The listing builds one solid part. Answer for the finished solid, in the listing's coordinates (mm). A direction names the side the tool comes from. Coordinates: 2 decimals unless noted, no trailing zeros. Loops run counter-clockwise (first coordinate to the right, second up) from the corner with the lowest first, then second, coordinate; pieces in that order, holes last. Notation, with made-up numbers: (42.25, 12.25) - (65.25, 12.25) arc R19 ccw to (65.25, 31.25) - close; hole circle Ø4 at (62, 44.25). An arc over 180 degrees is marked (long way). Return JSON: item names as keys, results as strings. Group by question number.
1. Section A-A (x = 125) is taken. Write down the section's boundary in (y, z) (3 decimals), and give its area (3 significant figures).
2. Find the intervals of material crossed by line 1 along X through (y, z) = (4.5, 0.75); line 2 along X through (y, z) = (-2.5, 0.75); line 3 along Y through (x, z) = (199, 0.25), in increasing order.
3. Which of the six approach directions +Z, -Z, +X, -X, +Y, -Y give full straight-line access (tool end or side, diameter ignored) to faces 1 (the face through (119.257, -4.588, 4.207)), 2 (the face through (22.92, -0.388, 2.955)), 3 (the face through (163.7, -0.1, -4.1))?
4. Each of these flat-tipped pins is pushed along its axis until it touches: P1, Ø2, axis at y = -5, z = -4.5, coming from the -X side; P2, Ø3, axis at x = 140, z = 3, coming from the +Y side; P3, Ø2, axis at x = 34, y = 4.5, coming from the +Z side; P4, Ø3, axis at x = 106, z = 0.5, coming from the +Y side. Where does it stop, or does it pass through?
5. The mould has two halves that part along X. Classify faces 4 (the face through (136.814, -3.135, -2.404)), 5 (the face through (69.702, -3.135, -2.404)), 6 (the face through (231.5, 3, 1)), 7 (the face through (260.162, -0.388, 2.955)): pulls with the +X half, pulls with the -X half, needs draft (parallel to the pull), parting line crosses it, or undercut.
```python
from build123d import *


with BuildPart() as part:
    # Esquisse1 → Révolution1 (revolve)
    with BuildSketch(Plane.XY):
        Polygon((0, 0), (0, 2.98), (1.7, 2.98), (1.7, 2.35), (3.4, 2.35), (3.4, 2.98), (41.9, 2.98), (41.9, 6.225), (65.9, 6.225), (65.9, 3.95), (73.4, 3.95), (73.4, 6.225), (97.4, 6.225), (97.4, 3.95), (109.7, 3.95), (109.7, 6.225), (128.55, 6.225), (128.55, 3.95), (144.85, 3.95), (144.85, 6.225), (163.7, 6.225), (163.7, 3.95), (176, 3.95), (176, 6.225), (200, 6.225), (200, 3.95), (207.5, 3.95), (207.5, 6.225), (231.5, 6.225), (231.5, 2.98), (257.6, 2.98), (257.6, 2.35), (259.3, 2.35), (259.3, 2.98), (261, 2.98), (261, 0), align=None)
    revolve(axis=Axis((0, 0, 0), (1, 0, 0)))


solid = part.part
```
The answers:
{
 "1": {"outline": "circle Ø12.45 at (0, 0)", "area": "122 mm2"},
 "2": {"line 1": "x = 41.9 to 65.9, 73.4 to 97.4, 109.7 to 128.55, 144.85 to 163.7, 176 to 200, 207.5 to 231.5", "line 2": "x = 0 to 1.7, 3.4 to 257.6, 259.3 to 261", "line 3": "y = -6.22 to 6.22"},
 "3": {"face 1": "+X, -X", "face 2": "-X", "face 3": "none"},
 "4": {"P1": "stops at x = 41.9", "P2": "stops at y = 3.65", "P3": "passes through", "P4": "stops at y = 3.95"},
 "5": {"face 4": "undercut", "face 5": "undercut", "face 6": "pulls with the +X half", "face 7": "needs draft"}
}
